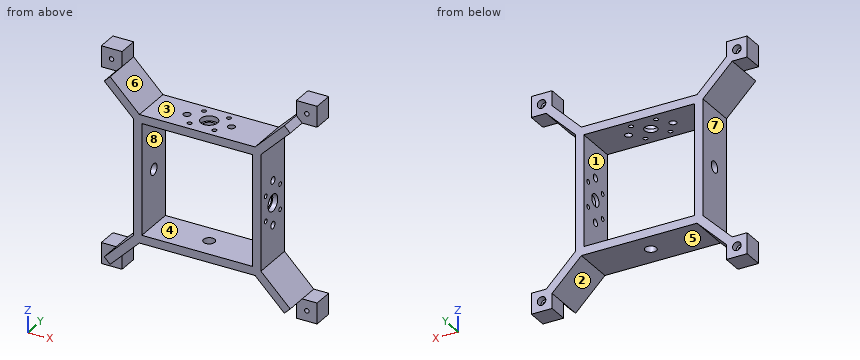
```python
from build123d import *

# Parameters (mm, degrees)
SKETCH_1_W               = 80
SKETCH_1_H               = 80
EXTRUDE_1_DEPTH          = 30
CUT_EXTRUDE_1_DEPTH      = 15
SKETCH_3_R               = 1.6
CUT_EXTRUDE_2_DEPTH      = 115.178894722
SKETCH_4_R               = 3.1
CUT_EXTRUDE_3_DEPTH      = 5
PATTERN_CIRCULAR_1_COUNT = 4
SKETCH_6_R               = 6.05
CUT_EXTRUDE_4_DEPTH      = 3.6
SKETCH_7_R               = 4.5
CUT_EXTRUDE_5_DEPTH      = 2.5
SKETCH_8_R               = 2.55
CUT_EXTRUDE_6_DEPTH      = 6
SKETCH_9_R               = 1.6
CUT_EXTRUDE_7_DEPTH      = 6
PATTERN_CIRCULAR_2_COUNT = 2
PATTERN_CIRCULAR_2_ANGLE = 90
SKETCH_10_R              = 4.05
CUT_EXTRUDE_8_DEPTH      = 6
PATTERN_CIRCULAR_3_COUNT = 2
PATTERN_CIRCULAR_3_ANGLE = 90
CUT_EXTRUDE_9_DEPTH      = 0.5


with BuildPart() as part:
    # 草图1 → 凸台-拉伸1 (new body)
    with BuildSketch(Plane(origin=(0, 0, 0), x_dir=(1, 0, 0), z_dir=(0, 1, 0))):
        Polygon((-77.9, 77.9), (-62.9, 77.9), (-62.9, 67.142640687), (-41.757359313, 46), (41.757359313, 46), (62.9, 67.142640687), (62.9, 77.9), (77.9, 77.9), (77.9, 62.9), (67.142640687, 62.9), (46, 41.757359313), (46, -41.757359313), (67.142640687, -62.9), (77.9, -62.9), (77.9, -77.9), (62.9, -77.9), (62.9, -67.142640687), (41.757359313, -46), (-41.757359313, -46), (-62.9, -67.142640687), (-62.9, -77.9), (-77.9, -77.9), (-77.9, -62.9), (-67.142640687, -62.9), (-46, -41.757359313), (-46, 41.757359313), (-67.142640687, 62.9), (-77.9, 62.9), align=None)
        Rectangle(SKETCH_1_W, SKETCH_1_H, mode=Mode.SUBTRACT)
    extrude(amount=EXTRUDE_1_DEPTH)

    # 草图2 → 切除-拉伸1 (cut)
    with BuildSketch(Plane(origin=(0, 0, 0), x_dir=(1, 0, 0), z_dir=(0, 1, 0))):
        Polygon((-77.9, 77.9), (-62.9, 77.9), (-62.9, 67.142640687), (-67.142640687, 62.9), (-77.9, 62.9), align=None)
        Polygon((62.9, 77.9), (77.9, 77.9), (77.9, 62.9), (67.142640687, 62.9), (62.9, 67.142640687), align=None)
        Polygon((77.9, -62.9), (77.9, -77.9), (62.9, -77.9), (62.9, -67.142640687), (67.142640687, -62.9), align=None)
        Polygon((-62.9, -77.9), (-77.9, -77.9), (-77.9, -62.9), (-67.142640687, -62.9), (-62.9, -67.142640687), align=None)
    extrude(amount=CUT_EXTRUDE_1_DEPTH, mode=Mode.SUBTRACT)

    # 草图3 → 切除-拉伸2 (cut, through all)
    with BuildSketch(Plane(origin=(0, 30, 0), x_dir=(1, 0, 0), z_dir=(0, 1, 0))):
        with Locations(Location((-70.5, 70.5, 0), (0, 0, 270))):
            Circle(SKETCH_3_R)
    cut_extrude_2 = extrude(amount=-CUT_EXTRUDE_2_DEPTH, mode=Mode.SUBTRACT)

    # 草图4 → 切除-拉伸3 (cut)
    with BuildSketch(Plane(origin=(0, 30, 0), x_dir=(1, 0, 0), z_dir=(0, 1, 0))):
        with Locations(Location((-70.5, 70.5, 0), (0, 0, 270))):
            Circle(SKETCH_4_R)
    cut_extrude_3 = extrude(amount=-CUT_EXTRUDE_3_DEPTH, mode=Mode.SUBTRACT)

    # 阵列(圆周)1: 切除-拉伸2, 切除-拉伸3 ×4 about axis
    pattern_circular_1_axis = Axis((0, 0, 0), (0, 1, 0))
    add([cut_extrude_2.rotate(pattern_circular_1_axis, i * 360 / PATTERN_CIRCULAR_1_COUNT) for i in range(1, PATTERN_CIRCULAR_1_COUNT)], mode=Mode.SUBTRACT)
    add([cut_extrude_3.rotate(pattern_circular_1_axis, i * 360 / PATTERN_CIRCULAR_1_COUNT) for i in range(1, PATTERN_CIRCULAR_1_COUNT)], mode=Mode.SUBTRACT)

    # 草图6 → 切除-拉伸4 (cut)
    with BuildSketch(Plane.XY.offset(46)):
        with Locations((0, 15)):
            Circle(SKETCH_6_R)
    cut_extrude_4 = extrude(amount=-CUT_EXTRUDE_4_DEPTH, mode=Mode.SUBTRACT)

    # 草图7 → 切除-拉伸5 (cut)
    with BuildSketch(Plane.XY.offset(42.4)):
        with Locations((0, 15)):
            Circle(SKETCH_7_R)
    cut_extrude_5 = extrude(amount=-CUT_EXTRUDE_5_DEPTH, mode=Mode.SUBTRACT)

    # 草图8 → 切除-拉伸6 (cut)
    with BuildSketch(Plane.XY.offset(46)):
        with Locations((-16, 15)):
            Circle(SKETCH_8_R)
        with Locations(Location((16, 15, 0), (0, 0, 180))):
            Circle(SKETCH_8_R)
    cut_extrude_6 = extrude(amount=-CUT_EXTRUDE_6_DEPTH, mode=Mode.SUBTRACT)

    # 草图9 → 切除-拉伸7 (cut)
    with BuildSketch(Plane.XY.offset(46)):
        with Locations((9, 24)):
            Circle(SKETCH_9_R)
        with Locations((9, 6)):
            Circle(SKETCH_9_R)
        with Locations((-9, 6)):
            Circle(SKETCH_9_R)
        with Locations((-9, 24)):
            Circle(SKETCH_9_R)
    cut_extrude_7 = extrude(amount=-CUT_EXTRUDE_7_DEPTH, mode=Mode.SUBTRACT)

    # 阵列(圆周)2: 切除-拉伸4, 切除-拉伸5, 切除-拉伸6, 切除-拉伸7 ×2 about axis
    pattern_circular_2_axis = Axis((0, 0, 0), (0, 1, 0))
    add([cut_extrude_4.rotate(pattern_circular_2_axis, i * PATTERN_CIRCULAR_2_ANGLE / (PATTERN_CIRCULAR_2_COUNT - 1)) for i in range(1, PATTERN_CIRCULAR_2_COUNT)], mode=Mode.SUBTRACT)
    add([cut_extrude_5.rotate(pattern_circular_2_axis, i * PATTERN_CIRCULAR_2_ANGLE / (PATTERN_CIRCULAR_2_COUNT - 1)) for i in range(1, PATTERN_CIRCULAR_2_COUNT)], mode=Mode.SUBTRACT)
    add([cut_extrude_6.rotate(pattern_circular_2_axis, i * PATTERN_CIRCULAR_2_ANGLE / (PATTERN_CIRCULAR_2_COUNT - 1)) for i in range(1, PATTERN_CIRCULAR_2_COUNT)], mode=Mode.SUBTRACT)
    add([cut_extrude_7.rotate(pattern_circular_2_axis, i * PATTERN_CIRCULAR_2_ANGLE / (PATTERN_CIRCULAR_2_COUNT - 1)) for i in range(1, PATTERN_CIRCULAR_2_COUNT)], mode=Mode.SUBTRACT)

    # 草图10 → 切除-拉伸8 (cut)
    with BuildSketch(Plane.ZY.offset(46)):
        with Locations((0, 15)):
            Circle(SKETCH_10_R)
    cut_extrude_8 = extrude(amount=-CUT_EXTRUDE_8_DEPTH, mode=Mode.SUBTRACT)

    # 阵列(圆周)3: 切除-拉伸8 ×2 about axis
    pattern_circular_3_axis = Axis((0, 0, 0), (0, -1, 0))
    for i in range(1, PATTERN_CIRCULAR_3_COUNT):
        add(cut_extrude_8.rotate(pattern_circular_3_axis, i * PATTERN_CIRCULAR_3_ANGLE / (PATTERN_CIRCULAR_3_COUNT - 1)), mode=Mode.SUBTRACT)

    # 草图11 → 切除-拉伸9 (cut)
    with BuildSketch(Plane(origin=(0, 30, 0), x_dir=(1, 0, 0), z_dir=(0, 1, 0))):
        Polygon((-77.9, 77.9), (-77.9, 62.9), (-67.142640687, 62.9), (-46, 41.757359313), (-46, -41.757359313), (-67.142640687, -62.9), (-77.9, -62.9), (-77.9, -77.9), (-62.9, -77.9), (-62.9, -67.142640687), (-41.757359313, -46), (41.757359313, -46), (62.9, -67.142640687), (62.9, -77.9), (77.9, -77.9), (77.9, -62.9), (67.142640687, -62.9), (46, -41.757359313), (46, 41.757359313), (67.142640687, 62.9), (77.9, 62.9), (77.9, 77.9), (62.9, 77.9), (62.9, 67.142640687), (41.757359313, 46), (-41.757359313, 46), (-62.9, 67.142640687), (-62.9, 77.9), align=None)
    extrude(amount=-CUT_EXTRUDE_9_DEPTH, mode=Mode.SUBTRACT)


solid = part.part
```
Check sheet for the modelled part. Datum: model origin and axes. Units: mm. Face numbers are marked on the shaded views. A direction names the side the tool comes from. Round coordinates to 2 decimals unless told otherwise and drop trailing zeros. Loops run counter-clockwise (first coordinate to the right, second up) from the corner with the lowest first, then second, coordinate; pieces in that order, holes last. Notation, with made-up numbers: (76.25, 17) -> (98.25, 17) arc R21 ccw to (98.25, 43) -> close; hole circle Ø1 at (84, 51.5). An arc over 180 degrees is marked (long way). Write item = value, one per line. Start each with the question number.
1) Sectioned sample at C-C, the plane x = 0. Record the cut outline in (y, z).
2) Sectioned sample at A-A, the plane x = 26. Record the cut outline in (y, z), plus the area to 3 significant figures.
3) Sectioned sample at B-B, the plane z = 16. Record the cut outline in (x, y), plus the area to 3 significant figures.
4) Set-up check for the marked faces 5, 6, 7 and 8: record each of +Z, -Z, +X, -X, +Y, -Y from which the full face is reachable in a straight line by a thin tool's end or side.
5) Sectioned sample at D-D, the plane z = 56. Record the cut outline in (x, y), plus the area to 3 significant figures.
6) Release check for a two-part mould opening along Z. For the marked faces 1, 2, 3 and 4 record: released by +Z, released by -Z, zero draft, split by the parting line, or undercut.
7) Thickness scan on probe 1 along Z at (x, y) = (70.5, 22.75); probe 2 along Y at (x, z) = (-16, 42.9); probe 3 along X at (y, z) = (19.5, 22.5). Record the ranges inside material, lowest first.
8) Gauge pin test, flat ends, axial feed: pin 1 Ø10 at (x, z) = (70.5, -70.5) entering from -Y; pin 2 Ø1.5 at (y, z) = (15, 5.5) entering from +X; pin 3 Ø9 at (y, z) = (14.5, 19.5) entering from -X. Record the tip position at first contact, or that the pin passes through.
Results are:
q1.outline = (0, -46) -> (10.95, -46) -> (10.95, -40) -> (0, -40) -> close; (0, 40) -> (10.5, 40) -> (10.5, 42.4) -> (8.95, 42.4) -> (8.95, 46) -> (0, 46) -> close; (19.05, -46) -> (29.5, -46) -> (29.5, -40) -> (19.05, -40) -> close; (19.5, 40) -> (29.5, 40) -> (29.5, 46) -> (21.05, 46) -> (21.05, 42.4) -> (19.5, 42.4) -> close
q2.outline = (0, -46) -> (29.5, -46) -> (29.5, -40) -> (0, -40) -> close; (0, 40) -> (29.5, 40) -> (29.5, 46) -> (0, 46) -> close
q2.area = 354 mm^2
q3.outline = (-46, 0) -> (-40, 0) -> (-40, 29.5) -> (-46, 29.5) -> close; (40, 0) -> (46, 0) -> (46, 12.45) -> (40, 12.45) -> close; (40, 17.55) -> (46, 17.55) -> (46, 29.5) -> (40, 29.5) -> close
q3.area = 323 mm^2
q4.face_5 = -Z, +Y, -Y
q4.face_6 = +Z, +Y, -Y
q4.face_7 = -X, +Y, -Y
q4.face_8 = +Y, -Y
q5.outline = (-60.24, 0) -> (-51.76, 0) -> (-51.76, 29.5) -> (-60.24, 29.5) -> close; (51.76, 0) -> (60.24, 0) -> (60.24, 29.5) -> (51.76, 29.5) -> close
q5.area = 501 mm^2
q6.face_1 = undercut
q6.face_2 = released by -Z
q6.face_3 = released by +Z
q6.face_4 = undercut
q7.probe_1 = -77.9 to -72.1, -68.9 to -62.9, 62.9 to 68.9, 72.1 to 77.9
q7.probe_2 = 0 to 12.45, 17.55 to 29.5
q7.probe_3 = -46 to -40, 40 to 46
q8.pin_1 = 15
q8.pin_2 = 46
q8.pin_3 = -46
